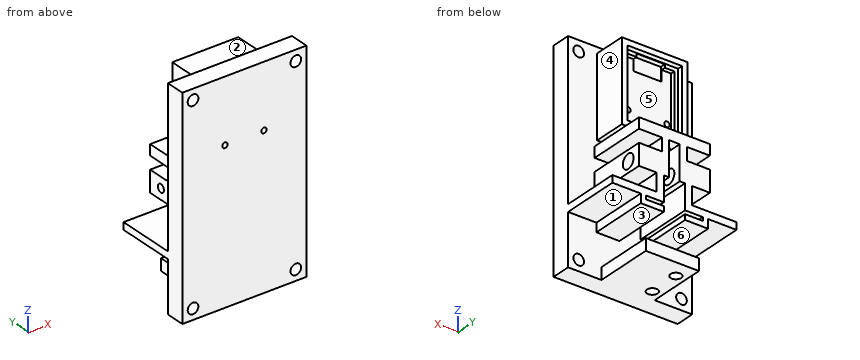
```python
from build123d import *

# Parameters (mm, degrees)
SKETCH1_W                      = 35
SKETCH1_H                      = 60
FLATBASE_DEPTH                 = 5.39
SKETCH19_R                     = 1.5
FLATBASEHOLES_DEPTH            = 6.39
SKETCH2_W                      = 20
SKETCH2_H                      = 3
FILAMENT_LASER_INTERFACE_DEPTH = 16.46
SKETCH4_R                      = 1.5
LASERHOLE_DEPTH                = 3
SKETCH8_W                      = 18.6
SKETCH8_H                      = 22.56
LASER_BASE_DEPTH               = 7.66
SKETCH9_W                      = 13.4
SKETCH9_H                      = 17.36
LASERBOARDMAINCUT_DEPTH        = 1.2
SKETCH11_W                     = 8
SKETCH11_H                     = 4
LASERBOARD_PINHPLES_DEPTH      = 1.5
SKETCH13_W                     = 18.6
SKETCH13_H                     = 22.56
SKETCH13_W_2                   = 15.5
SKETCH13_H_2                   = 19.46
LASERBOARD_SKIRTING_DEPTH      = 1.5
SKETCH14_R                     = 0.75
LASERBOARD_SCREWHOLES_DEPTH    = 12.85
SKETCH20_W                     = 20
SKETCH20_H                     = 6
BOSS_EXTRUDE1_DEPTH            = 16.46
SKETCH22_R                     = 1.115
CUT_EXTRUDE1_DEPTH             = 20
SKETCH23_W                     = 3
SKETCH23_H                     = 6
CUT_EXTRUDE2_DEPTH             = 10
SKETCH24_R                     = 2
CUT_EXTRUDE3_DEPTH             = 4
SKETCH25_R                     = 2
CUT_EXTRUDE4_DEPTH             = 4
SKETCH26_W                     = 2
SKETCH26_H                     = 3.623584384
BOSS_EXTRUDE2_DEPTH            = 16.46
SKETCH27_W                     = 15
SKETCH27_H                     = 3.326415616
BOSS_EXTRUDE3_DEPTH            = 16.46
SKETCH28_R                     = 1.5
CUT_EXTRUDE5_DEPTH             = 3.326416
BOSS_EXTRUDE4_DEPTH            = 16.46


with BuildPart() as part:
    # Sketch1 → FlatBase (new body)
    with BuildSketch(Plane(origin=(0, 0, 0), x_dir=(1, 0, 0), z_dir=(0, 1, 0))):
        Rectangle(SKETCH1_W, SKETCH1_H)
    extrude(amount=FLATBASE_DEPTH)

    # Sketch19 → FlatBaseHoles (cut, through all)
    with BuildSketch(Plane(origin=(0, 5.39, 0), x_dir=(1, 0, 0), z_dir=(0, 1, 0))):
        with Locations((-14.5, 27)):
            Circle(SKETCH19_R)
        with Locations((14.5, 27)):
            Circle(SKETCH19_R)
        with Locations((14.5, -27)):
            Circle(SKETCH19_R)
        with Locations((-14.5, -27)):
            Circle(SKETCH19_R)
    extrude(amount=-FLATBASEHOLES_DEPTH, mode=Mode.SUBTRACT)

    # Sketch2 → Filament-Laser-Interface (add)
    with BuildSketch(Plane(origin=(0, 5.39, 0), x_dir=(1, 0, 0), z_dir=(0, 1, 0))):
        with Locations((0, -2.5)):
            Rectangle(SKETCH2_W, SKETCH2_H)
    extrude(amount=FILAMENT_LASER_INTERFACE_DEPTH)

    # Sketch4 → LaserHole (cut)
    with BuildSketch(Plane(origin=(0, 0, 1), x_dir=(-1, 0, 0), z_dir=(0, 0, -1))):
        with Locations((0, 17.85)):
            Circle(SKETCH4_R)
    extrude(amount=-LASERHOLE_DEPTH, mode=Mode.SUBTRACT)

    # Sketch8 → Laser-Base (add)
    with BuildSketch(Plane(origin=(0, 5.39, 0), x_dir=(1, 0, 0), z_dir=(0, 1, 0))):
        with Locations((0, -17.07)):
            Rectangle(SKETCH8_W, SKETCH8_H)
    extrude(amount=LASER_BASE_DEPTH)

    # Sketch9 → LaserBoardMainCut (cut)
    with BuildSketch(Plane(origin=(0, 13.05, 0), x_dir=(1, 0, 0), z_dir=(0, 1, 0))):
        with Locations((0, -17.07)):
            Rectangle(SKETCH9_W, SKETCH9_H)
    extrude(amount=-LASERBOARDMAINCUT_DEPTH, mode=Mode.SUBTRACT)

    # Sketch11 → LaserBoard-PinHples (cut)
    with BuildSketch(Plane(origin=(0, 13.05, 0), x_dir=(1, 0, 0), z_dir=(0, 1, 0))):
        with Locations((0, -24.65)):
            Rectangle(SKETCH11_W, SKETCH11_H)
    extrude(amount=-LASERBOARD_PINHPLES_DEPTH, mode=Mode.SUBTRACT)

    # Sketch13 → LaserBoard-Skirting (add)
    with BuildSketch(Plane(origin=(0, 13.05, 0), x_dir=(1, 0, 0), z_dir=(0, 1, 0))):
        with Locations((0, -17.07)):
            Rectangle(SKETCH13_W, SKETCH13_H)
        with Locations((0, -17.07)):
            Rectangle(SKETCH13_W_2, SKETCH13_H_2, mode=Mode.SUBTRACT)
    extrude(amount=LASERBOARD_SKIRTING_DEPTH)

    # Sketch14 → LaserBoard-ScrewHoles (cut, through all)
    with BuildSketch(Plane(origin=(0, 11.85, 0), x_dir=(1, 0, 0), z_dir=(0, 1, 0))):
        with Locations((5.5, -12.17)):
            Circle(SKETCH14_R)
        with Locations((-5.5, -12.17)):
            Circle(SKETCH14_R)
    extrude(amount=-LASERBOARD_SCREWHOLES_DEPTH, mode=Mode.SUBTRACT)

    # Sketch20 → Boss-Extrude1 (add)
    with BuildSketch(Plane(origin=(0, 5.39, 0), x_dir=(1, 0, 0), z_dir=(0, 1, 0))):
        with Locations((0, 5.623584384)):
            Rectangle(SKETCH20_W, SKETCH20_H)
    extrude(amount=BOSS_EXTRUDE1_DEPTH)

    # Sketch22 → Cut-Extrude1 (cut)
    with BuildSketch(Plane(origin=(10, 0, 0), x_dir=(0, 0, -1), z_dir=(1, 0, 0))):
        with Locations((5.623584384, 17.85)):
            Circle(SKETCH22_R)
    extrude(amount=-CUT_EXTRUDE1_DEPTH, mode=Mode.SUBTRACT)

    # Sketch23 → Cut-Extrude2 (cut)
    with BuildSketch(Plane(origin=(0, 21.85, 0), x_dir=(1, 0, 0), z_dir=(0, 1, 0))):
        with Locations((0, 5.623584384)):
            Rectangle(SKETCH23_W, SKETCH23_H)
    extrude(amount=-CUT_EXTRUDE2_DEPTH, mode=Mode.SUBTRACT)

    # Sketch24 → Cut-Extrude3 (cut)
    with BuildSketch(Plane(origin=(10, 0, 0), x_dir=(0, 0, -1), z_dir=(1, 0, 0))):
        with Locations((5.623584384, 17.85)):
            Circle(SKETCH24_R)
    extrude(amount=-CUT_EXTRUDE3_DEPTH, mode=Mode.SUBTRACT)

    # Sketch25 → Cut-Extrude4 (cut)
    with BuildSketch(Plane(origin=(-1.5, 0, 0), x_dir=(0, 0, -1), z_dir=(1, 0, 0))):
        with Locations((5.623584384, 17.85)):
            Circle(SKETCH25_R)
    extrude(amount=-CUT_EXTRUDE4_DEPTH, mode=Mode.SUBTRACT)

    # Sketch26 → Boss-Extrude2 (add)
    with BuildSketch(Plane(origin=(0, 5.39, 0), x_dir=(1, 0, 0), z_dir=(0, 1, 0))):
        with Locations((2.5, 0.811792192)):
            Rectangle(SKETCH26_W, SKETCH26_H)
        with Locations((-2.5, 0.811792192)):
            Rectangle(SKETCH26_W, SKETCH26_H)
    extrude(amount=BOSS_EXTRUDE2_DEPTH)

    # Sketch27 → Boss-Extrude3 (add)
    with BuildSketch(Plane(origin=(0, 5.39, 0), x_dir=(1, 0, 0), z_dir=(0, 1, 0))):
        with Locations((0.585, 28.336792192)):
            Rectangle(SKETCH27_W, SKETCH27_H)
    extrude(amount=BOSS_EXTRUDE3_DEPTH)

    # Sketch28 → Cut-Extrude5 (cut)
    with BuildSketch(Plane.XY.offset(-26.673584384)):
        with Locations((-4.145, 8.195)):
            Circle(SKETCH28_R)
        with Locations((-4.145, 16.945)):
            Circle(SKETCH28_R)
    extrude(amount=-CUT_EXTRUDE5_DEPTH, mode=Mode.SUBTRACT)

    # Sketch29 → Boss-Extrude4 (add)
    with BuildSketch(Plane(origin=(0, 5.39, 0), x_dir=(1, 0, 0), z_dir=(0, 1, 0))):
        Polygon((-17.5, 15.623584384), (-9.5, 15.623584384), (-9.5, 18.123584384), (-3, 18.123584384), (-3, 16.623584384), (-8, 16.623584384), (-8, 15.623584384), (-3, 15.623584384), (-3, 13.623584384), (-3, 8.623584384), (-5, 8.623584384), (-5, 13.623584384), (-17.5, 13.623584384), align=None)
        Polygon((17.5, 15.623584384), (17.5, 13.623584384), (5, 13.623584384), (5, 8.623584384), (3, 8.623584384), (3, 13.623584384), (3, 15.623584384), (8, 15.623584384), (8, 16.623584384), (3, 16.623584384), (3, 18.123584384), (9.5, 18.123584384), (9.5, 15.623584384), align=None)
    extrude(amount=BOSS_EXTRUDE4_DEPTH)


solid = part.part
```
Read the model definition and answer for the solid it produces. Units are mm, in the model's axes. Face numbers are marked on the shaded views. A direction names the side the tool comes from. Round coordinates to 2 decimals unless told otherwise and drop trailing zeros. Write each loop counter-clockwise with the first axis right and the second up, starting at its lowest first coordinate (ties: lowest second). Pieces come first, ordered by that corner, then holes. Notation, with made-up numbers: M -18,65.25 L -2,65.25 A33 cw -2,100.25 Z; hole C 16,-9.75 d10. An arc over 180 degrees is marked long. One line per item, written item: value.
Q1. Find section B-B on z = 12.17. Write down the section's boundary in (x, y), plus the area to 3 significant figures.
Data:
outline: M -17.5,0 L -6.25,0 L -6.25,11.85 L -6.7,11.85 L -6.7,13.05 L -7.75,13.05 L -7.75,14.55 L -9.3,14.55 L -9.3,5.39 L -17.5,5.39 Z; M -4.75,0 L 4.75,0 L 4.75,11.85 L -4.75,11.85 Z; M 6.25,0 L 17.5,0 L 17.5,5.39 L 9.3,5.39 L 9.3,14.55 L 7.75,14.55 L 7.75,13.05 L 6.7,13.05 L 6.7,11.85 L 6.25,11.85 Z
area: 284 mm2
Q2. Find section C-C on x = -14.5. Write down the section's boundary in (y, z), plus the area to 3 significant figures.
Data:
outline: M 0,-30 L 5.39,-30 L 5.39,-28.5 L 0,-28.5 Z; M 0,-25.5 L 5.39,-25.5 L 5.39,-15.62 L 21.85,-15.62 L 21.85,-13.62 L 5.39,-13.62 L 5.39,25.5 L 0,25.5 Z; M 0,28.5 L 5.39,28.5 L 5.39,30 L 0,30 Z
area: 324 mm2
Q3. Straight lines are drawn through the part: line 1 (Z direction, x = 14.5, y = 3.15); line 2 (X direction, y = 7, z = 12.17); line 3 (Z direction, x = 9, y = 15.25). For each, find the intervals that lie inside material, in ascending order. Write a range as [from, to].
Data:
line 1: [-30, -28.5], [-25.5, 25.5], [28.5, 30]
line 2: [-9.3, -6.25], [-4.75, 4.75], [6.25, 9.3]
line 3: [-18.12, -13.62], [-8.62, -2.62], [1, 4]
Q4. Find section D-D on y = 4.5. Write down the section's boundary in (x, z).
Data:
outline: M -17.5,-30 L 17.5,-30 L 17.5,30 L -17.5,30 Z; hole C -14.5,-27 d3; hole C -14.5,27 d3; hole C -5.5,12.17 d1.5; hole C 5.5,12.17 d1.5; hole C 14.5,-27 d3; hole C 14.5,27 d3
Q5. Flat-ended cylindrical pins translate along their axes: pin 1 Ø1 at (y, z) = (17.5, -9) entering from +X; pin 2 Ø8 at (y, z) = (18, 22) entering from -X; pin 3 Ø5 at (x, z) = (13, -20.5) entering from +Y; pin 4 Ø5.5 at (y, z) = (11.5, -11.5) entering from -X. Find the tip coordinate at first contact, or state that the pin passes through.
Data:
pin 1: x = 10
pin 2: x = -9.3
pin 3: y = 5.39
pin 4: x = -17.5
Q6. Which of the six approach directions +Z, -Z, +X, -X, +Y, -Y give full straight-line access (tool end or side, diameter ignored) to the marked faces 1, 2 and 3?
Data:
face 1: -Z, +X, +Y
face 2: +Z, +X, -X, +Y
face 3: +X, -X, +Y
Q7. For a pull along X with two mould halves and no side action, classify the marked faces 4, 5 and 6 as +X half, -X half, draft (parallel to the pull), parting line (faces both ways), or undercut.
Data:
face 4: +X half
face 5: undercut
face 6: draft
